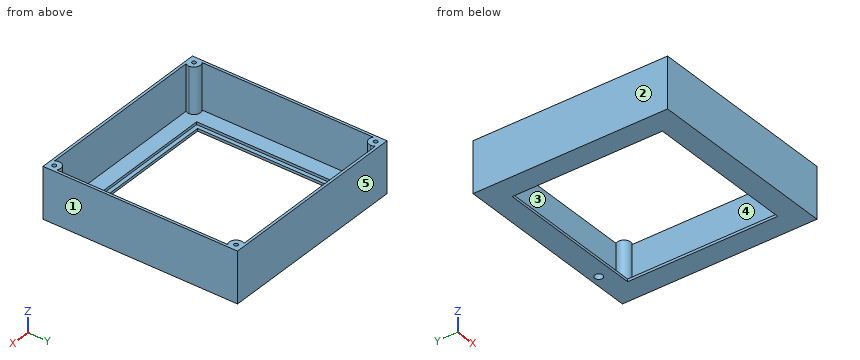
```python
from build123d import *

# Parameters (mm, degrees)
F1_DEPTH = 4
F0_W     = 115
F0_H     = 3
F0_W_2   = 3
F0_H_2   = 115
F2_DEPTH = 2
F3_R     = 3
F4_DEPTH = 4
F5_W     = 149
F5_H     = 149
F6_DEPTH = 35
F7_R     = 1.5
F8_DEPTH = 35


with BuildPart() as f1:
    # F0 (on Top) → F1 (new body)
    with BuildSketch(Plane.XY):
        Polygon((74.5, 74.5), (60.5, 74.5), (-60.5, 74.5), (-74.5, 74.5), (-74.5, 60.5), (-74.5, -60.5), (-74.5, -74.5), (-60.5, -74.5), (60.5, -74.5), (74.5, -74.5), (74.5, -60.5), (74.5, 60.5), align=None)
        Polygon((57.5, 60.5), (60.5, 60.5), (60.5, 57.5), (60.5, -57.5), (60.5, -60.5), (57.5, -60.5), (-57.5, -60.5), (-60.5, -60.5), (-60.5, -57.5), (-60.5, 57.5), (-60.5, 60.5), (-57.5, 60.5), align=None, mode=Mode.SUBTRACT)
    extrude(amount=F1_DEPTH)

    # F0 (on Top) → F2 (join)
    with BuildSketch(Plane.XY):
        with Locations((0, 59)):
            Rectangle(F0_W, F0_H)
        with Locations((59, 59)):
            Rectangle(F0_W_2, F0_H)
        with Locations((59, 0)):
            Rectangle(F0_W_2, F0_H_2)
        with Locations((59, -59)):
            Rectangle(F0_W_2, F0_H)
        with Locations((0, -59)):
            Rectangle(F0_W, F0_H)
        with Locations((-59, 0)):
            Rectangle(F0_W_2, F0_H_2)
        with Locations((-59, -59)):
            Rectangle(F0_W_2, F0_H)
        with Locations((-59, 59)):
            Rectangle(F0_W_2, F0_H)
    extrude(amount=F2_DEPTH)

    # F3 (on face) → F4 (cut, through all)
    with BuildSketch(Plane.XY.offset(4)):
        with Locations((42.5219088793, 68.0854469538)):
            Circle(F3_R)
    extrude(amount=-F4_DEPTH, mode=Mode.SUBTRACT)

    # F5 (on face) → F6 (join)
    with BuildSketch(Plane.XY.offset(4)):
        Rectangle(F5_W, F5_H)
        Polygon((-60.5, 72.5), (60.5, 72.5), (72.5, 72.5), (72.5, 60.5), (72.5, -60.5), (72.5, -72.5), (60.5, -72.5), (-60.5, -72.5), (-72.5, -72.5), (-72.5, -60.5), (-72.5, 60.5), (-72.5, 72.5), align=None, mode=Mode.SUBTRACT)
    extrude(amount=F6_DEPTH)

    # F7 (on face) → F8 (join)
    with BuildSketch(Plane.XY.offset(39)):
        with BuildLine():
            ThreePointArc((-72.5, 65.5269179106), (-67.3087125968, 65.1559040438), (-64.6000009775, 69.6000009775))
            ThreePointArc((-64.6000009775, 69.6000009775), (-64.8373643478, 71.1222665039), (-65.5269179106, 72.5))
            Line((-65.5269179106, 72.5), (-72.5, 72.5))
            Line((-72.5, 72.5), (-72.5, 65.5269179106))
        make_face()
        with Locations((-69.6000009775, 69.6000009775)):
            Circle(F7_R, mode=Mode.SUBTRACT)
        with BuildLine():
            Line((72.5, 72.5), (65.5269179106, 72.5))
            ThreePointArc((65.5269179106, 72.5), (66.0644670716, 66.0644670716), (72.5, 65.5269179106))
            Line((72.5, 65.5269179106), (72.5, 72.5))
        make_face()
        with Locations((69.6000009775, 69.6000009775)):
            Circle(F7_R, mode=Mode.SUBTRACT)
        with BuildLine():
            Line((72.5, -72.5), (72.5, -65.5269179106))
            ThreePointArc((72.5, -65.5269179106), (66.0644670716, -66.0644670716), (65.5269179106, -72.5))
            Line((65.5269179106, -72.5), (72.5, -72.5))
        make_face()
        with Locations((69.6000009775, -69.6000009775)):
            Circle(F7_R, mode=Mode.SUBTRACT)
        with BuildLine():
            ThreePointArc((-64.6000009775, -69.6000009775), (-67.3087125968, -65.1559040438), (-72.5, -65.5269179106))
            Line((-72.5, -65.5269179106), (-72.5, -72.5))
            Line((-72.5, -72.5), (-65.5269179106, -72.5))
            ThreePointArc((-65.5269179106, -72.5), (-64.8373643478, -71.1222665039), (-64.6000009775, -69.6000009775))
        make_face()
        with Locations((-69.6000009775, -69.6000009775)):
            Circle(F7_R, mode=Mode.SUBTRACT)
    extrude(amount=-F8_DEPTH)


solid = f1.part
```
Part model, mm, in its own coordinate system. Face numbers are marked on the shaded views. A direction names the side the tool comes from. Give positions to 0.01 mm unless a question says otherwise; leave off trailing zeros. Write each loop counter-clockwise with the first axis right and the second up, starting at its lowest first coordinate (ties: lowest second). Pieces come first, ordered by that corner, then holes. Notation, with made-up numbers: M -19.5,-18 L 6.5,-18 A26 cw 6.5,4 Z; hole C 2.25,84.5 d1. An arc over 180 degrees is marked long. Use CSV: the item, a comma, the result in double quotes.
Item 1: Slice it at D-D on x = 41.5. Write the cut outline in (y, z).
Taken from the geometry:
outline,"M -74.5,0 L -57.5,0 L -57.5,2 L -60.5,2 L -60.5,4 L -72.5,4 L -72.5,39 L -74.5,39 Z; M 57.5,0 L 65.26,0 L 65.26,4 L 60.5,4 L 60.5,2 L 57.5,2 Z; M 70.91,0 L 74.5,0 L 74.5,39 L 72.5,39 L 72.5,4 L 70.91,4 Z"
Item 2: Drill centre lines: probe 1 along Y at (x, z) = (69.6, 12); probe 2 along Y at (x, z) = (31.5, 7). Where is each one in solid material? Low to high.
Taken from the geometry:
probe 1,"y = -74.5 to -71.1, -68.1 to -64.6, 64.6 to 68.1, 71.1 to 74.5"
probe 2,"y = -74.5 to -72.5, 72.5 to 74.5"
Item 3: Pin check, flat tips, straight feed: P1, Ø6, axis at x = -54, y = 57, coming from the +Z side; P2, Ø7, axis at x = 42.52, y = 68.09, coming from the -Z side; P3, Ø1.5, axis at x = 69, y = -69.5, coming from the +Z side. Stop position of each tip, or through.
Taken from the geometry:
P1,"stops at z = 2"
P2,"stops at z = 0"
P3,"stops at z = 4"
Item 4: Slice it at A-A on y = 39. Write the cut outline in (x, z).
Taken from the geometry:
outline,"M -74.5,0 L -57.5,0 L -57.5,2 L -60.5,2 L -60.5,4 L -72.5,4 L -72.5,39 L -74.5,39 Z; M 57.5,0 L 74.5,0 L 74.5,39 L 72.5,39 L 72.5,4 L 60.5,4 L 60.5,2 L 57.5,2 Z"
Item 5: Pull direction X, two halves, no side cores. Call the marked faces 1, 2 and 3: +X half, -X half, draft (parallel to the pull), parting line (faces both ways), or undercut.
Taken from the geometry:
face 1,"+X half"
face 2,"-X half"
face 3,"undercut"
Item 6: Which spindle directions (+Z, -Z, +X, -X, +Y, -Y) get a long thin tool onto all of the face, cutting with end or side? Do the marked faces 4 and 5. Say none if no direction does.
Taken from the geometry:
face 4,"+Z"
face 5,"+Z, -Z, +X, -X, +Y"
Item 7: Slice it at C-C on z = 24. Write the cut outline in (x, y), plus the area to 3 significant figures.
Taken from the geometry:
outline,"M -74.5,-74.5 L 74.5,-74.5 L 74.5,74.5 L -74.5,74.5 Z; hole M -72.5,-65.53 A5 cw -65.53,-72.5 L 65.53,-72.5 A5 cw 72.5,-65.53 L 72.5,65.53 A5 cw 65.53,72.5 L -65.53,72.5 A5 cw -72.5,65.53 Z; hole C -69.6,-69.6 d3; hole C -69.6,69.6 d3; hole C 69.6,-69.6 d3; hole C 69.6,69.6 d3"
area,"1,370 mm²"
